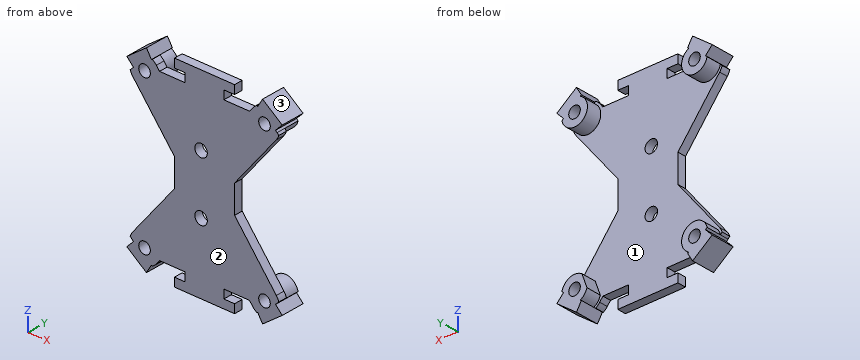
```python
from build123d import *

# Parameters (mm, degrees)
SKETCH1_R               = 24.07
BOSS_EXTRUDE1_DEPTH     = 2
BOSS_EXTRUDE2_DEPTH     = 5.5
BOSS_EXTRUDE5_REACH     = 36.482
SKETCH2_R               = 3
SKETCH1_5_R             = 34.31362745
CUT_EXTRUDE3_DEPTH      = 35.48158639
CUT_EXTRUDE3_DEPTH_BACK = 35.48158639
M2_5_CLEARANCE_HOLE1_D  = 2.7
CUT_EXTRUDE4_DEPTH      = 35.48158639
SKETCH10_R              = 1.45
CUT_EXTRUDE6_DEPTH      = 30.773984948
CUT_EXTRUDE7_DEPTH      = 3.5


with BuildPart() as part:
    # Sketch1 → Boss-Extrude1 (new body)
    with BuildSketch(Plane(origin=(0, 0, 0), x_dir=(1, 0, 0), z_dir=(0, 1, 0))):
        with Locations(Location((0, 0, 0), (0, 0, 270))):
            Circle(SKETCH1_R)
    extrude(amount=BOSS_EXTRUDE1_DEPTH)

    # Sketch1<3> → Boss-Extrude2 (add)
    with BuildSketch(Plane(origin=(0, 0, 0), x_dir=(1, 0, 0), z_dir=(0, 1, 0))):
        with BuildLine():
            ThreePointArc((12.366915807, 20.650043424), (14.541516735, 19.180959075), (16.543257949, 17.483864459))
            Line((16.543257949, 17.483864459), (18.089781085, 19.118318867))
            Line((18.089781085, 19.118318867), (13.523019488, 22.580483607))
            Line((13.523019488, 22.580483607), (12.366915807, 20.650043424))
        make_face()
        with BuildLine():
            ThreePointArc((16.543257949, -17.483864459), (14.541516735, -19.180959075), (12.366915807, -20.650043424))
            Line((12.366915807, -20.650043424), (13.523019488, -22.580483607))
            Line((13.523019488, -22.580483607), (18.089781085, -19.118318867))
            Line((18.089781085, -19.118318867), (16.543257949, -17.483864459))
        make_face()
        with BuildLine():
            ThreePointArc((-16.543257949, 17.483864459), (-14.541516735, 19.180959075), (-12.366915807, 20.650043424))
            Line((-12.366915807, 20.650043424), (-13.523019488, 22.580483607))
            Line((-13.523019488, 22.580483607), (-18.089781085, 19.118318867))
            Line((-18.089781085, 19.118318867), (-16.543257949, 17.483864459))
        make_face()
        with BuildLine():
            ThreePointArc((-12.366915807, -20.650043424), (-14.541516735, -19.180959075), (-16.543257949, -17.483864459))
            Line((-16.543257949, -17.483864459), (-18.089781085, -19.118318867))
            Line((-18.089781085, -19.118318867), (-13.523019488, -22.580483607))
            Line((-13.523019488, -22.580483607), (-12.366915807, -20.650043424))
        make_face()
    extrude(amount=BOSS_EXTRUDE2_DEPTH)

    # Boss-Extrude5: up to this face of the body (flat: up to its plane)
    boss_extrude5_end = Plane(part.part.faces().sort_by_distance((15.168468653, 5.5, 20.00793877))[0])
    # Sketch2 → Boss-Extrude5 (add, up to the picked face)
    with BuildSketch(Plane(origin=(0, 0, 0), x_dir=(1, 0, 0), z_dir=(0, 1, 0)), mode=Mode.PRIVATE) as boss_extrude5_sk1:
        with Locations((13.97, 17.78)):
            Circle(SKETCH2_R)
    boss_extrude5_tool1 = split(extrude(boss_extrude5_sk1.sketch, amount=BOSS_EXTRUDE5_REACH, mode=Mode.PRIVATE), bisect_by=boss_extrude5_end, keep=Keep.BOTH, mode=Mode.PRIVATE)
    # Sketch2 → Boss-Extrude5 (add, up to the picked face)
    with BuildSketch(Plane(origin=(0, 0, 0), x_dir=(1, 0, 0), z_dir=(0, 1, 0)), mode=Mode.PRIVATE) as boss_extrude5_sk2:
        with Locations((13.97, -17.78)):
            Circle(SKETCH2_R)
    boss_extrude5_tool2 = split(extrude(boss_extrude5_sk2.sketch, amount=BOSS_EXTRUDE5_REACH, mode=Mode.PRIVATE), bisect_by=boss_extrude5_end, keep=Keep.BOTH, mode=Mode.PRIVATE)
    # Sketch2 → Boss-Extrude5 (add, up to the picked face)
    with BuildSketch(Plane(origin=(0, 0, 0), x_dir=(1, 0, 0), z_dir=(0, 1, 0)), mode=Mode.PRIVATE) as boss_extrude5_sk3:
        with Locations((-13.97, -17.78)):
            Circle(SKETCH2_R)
    boss_extrude5_tool3 = split(extrude(boss_extrude5_sk3.sketch, amount=BOSS_EXTRUDE5_REACH, mode=Mode.PRIVATE), bisect_by=boss_extrude5_end, keep=Keep.BOTH, mode=Mode.PRIVATE)
    # Sketch2 → Boss-Extrude5 (add, up to the picked face)
    with BuildSketch(Plane(origin=(0, 0, 0), x_dir=(1, 0, 0), z_dir=(0, 1, 0)), mode=Mode.PRIVATE) as boss_extrude5_sk4:
        with Locations((-13.97, 17.78)):
            Circle(SKETCH2_R)
    boss_extrude5_tool4 = split(extrude(boss_extrude5_sk4.sketch, amount=BOSS_EXTRUDE5_REACH, mode=Mode.PRIVATE), bisect_by=boss_extrude5_end, keep=Keep.BOTH, mode=Mode.PRIVATE)
    add(boss_extrude5_tool1.solids().sort_by(Axis((13.97, 0, -17.78), (0, 1, 0)))[0])
    add(boss_extrude5_tool2.solids().sort_by(Axis((13.97, 0, 17.78), (0, 1, 0)))[0])
    add(boss_extrude5_tool3.solids().sort_by(Axis((-13.97, 0, 17.78), (0, 1, 0)))[0])
    add(boss_extrude5_tool4.solids().sort_by(Axis((-13.97, 0, -17.78), (0, 1, 0)))[0])

    # Sketch1<5> → Cut-Extrude3 (cut, two sides)
    with BuildSketch(Plane(origin=(0, 0, 0), x_dir=(1, 0, 0), z_dir=(0, 1, 0))) as cut_extrude3_sk:
        Circle(SKETCH1_5_R)
        with BuildLine():
            Line((18.089781085, 19.118318867), (16.543257949, 17.483864459))
            ThreePointArc((16.543257949, 17.483864459), (22.108382108, 9.517580605), (24.07, 0))
            ThreePointArc((24.07, 0), (22.108382108, -9.517580605), (16.543257949, -17.483864459))
            Line((16.543257949, -17.483864459), (18.089781085, -19.118318867))
            Line((18.089781085, -19.118318867), (13.523019488, -22.580483607))
            Line((13.523019488, -22.580483607), (12.366915807, -20.650043424))
            ThreePointArc((12.366915807, -20.650043424), (0, -24.07), (-12.366915807, -20.650043424))
            Line((-12.366915807, -20.650043424), (-13.523019488, -22.580483607))
            Line((-13.523019488, -22.580483607), (-18.089781085, -19.118318867))
            Line((-18.089781085, -19.118318867), (-16.543257949, -17.483864459))
            ThreePointArc((-16.543257949, -17.483864459), (-24.07, 0), (-16.543257949, 17.483864459))
            Line((-16.543257949, 17.483864459), (-18.089781085, 19.118318867))
            Line((-18.089781085, 19.118318867), (-13.523019488, 22.580483607))
            Line((-13.523019488, 22.580483607), (-12.366915807, 20.650043424))
            ThreePointArc((-12.366915807, 20.650043424), (0, 24.07), (12.366915807, 20.650043424))
            Line((12.366915807, 20.650043424), (13.523019488, 22.580483607))
            Line((13.523019488, 22.580483607), (18.089781085, 19.118318867))
        make_face(mode=Mode.SUBTRACT)
    extrude(amount=CUT_EXTRUDE3_DEPTH, mode=Mode.SUBTRACT)
    extrude(cut_extrude3_sk.sketch, amount=-CUT_EXTRUDE3_DEPTH_BACK, mode=Mode.SUBTRACT)

    # M2.5 Clearance Hole1 (through all)
    with Locations(Plane(origin=(0, 5.5, 0), x_dir=(1, 0, 0), z_dir=(0, 1, 0))):
        with Locations((-13.97, 17.78), (13.97, 17.78), (13.97, -17.78), (-13.97, -17.78)):
            Hole(M2_5_CLEARANCE_HOLE1_D / 2)

    # Sketch8 → Cut-Extrude4 (cut, through all)
    with BuildSketch(Plane.XZ):
        with BuildLine():
            ThreePointArc((-12.157407277, 20.77407876), (-11.650071144, 20.400673597), (-11.217885814, 19.942375432))
            Line((-11.217885814, 19.942375432), (-10.477447975, 19))
            Line((-10.477447975, 19), (-4.5, 19))
            Line((-4.5, 19), (-4.5, 21))
            Line((-4.5, 21), (-7, 21))
            Line((-7, 21), (-7, 23))
            Line((-7, 23), (7, 23))
            Line((7, 23), (7, 21))
            Line((7, 21), (4.5, 21))
            Line((4.5, 21), (4.5, 19))
            Line((4.5, 19), (10.477447975, 19))
            Line((10.477447975, 19), (11.217885814, 19.942375432))
            ThreePointArc((11.217885814, 19.942375432), (11.650071144, 20.400673597), (12.157407277, 20.77407876))
            ThreePointArc((12.157407277, 20.77407876), (0, 24.07), (-12.157407277, 20.77407876))
        make_face()
        with BuildLine():
            Line((7, 3.244024695), (7, -3.244024695))
            Line((7, -3.244024695), (16.722114186, -15.617624568))
            ThreePointArc((16.722114186, -15.617624568), (17.065148682, -16.145969817), (17.307920228, -16.727247155))
            ThreePointArc((17.307920228, -16.727247155), (24.07, 0), (17.307920228, 16.727247155))
            ThreePointArc((17.307920228, 16.727247155), (17.065148682, 16.145969817), (16.722114186, 15.617624568))
            Line((16.722114186, 15.617624568), (7, 3.244024695))
        make_face()
        with BuildLine():
            Line((-7, -3.244024695), (-7, 3.244024695))
            Line((-7, 3.244024695), (-16.722114186, 15.617624568))
            ThreePointArc((-16.722114186, 15.617624568), (-17.065148682, 16.145969817), (-17.307920228, 16.727247155))
            ThreePointArc((-17.307920228, 16.727247155), (-24.07, 0), (-17.307920228, -16.727247155))
            ThreePointArc((-17.307920228, -16.727247155), (-17.065148682, -16.145969817), (-16.722114186, -15.617624568))
            Line((-16.722114186, -15.617624568), (-7, -3.244024695))
        make_face()
        with BuildLine():
            Line((11.217885814, -19.942375432), (10.477447975, -19))
            Line((10.477447975, -19), (4.5, -19))
            Line((4.5, -19), (4.5, -21))
            Line((4.5, -21), (7, -21))
            Line((7, -21), (7, -23))
            Line((7, -23), (-7, -23))
            Line((-7, -23), (-7, -21))
            Line((-7, -21), (-4.5, -21))
            Line((-4.5, -21), (-4.5, -19))
            Line((-4.5, -19), (-10.477447975, -19))
            Line((-10.477447975, -19), (-11.217885814, -19.942375432))
            ThreePointArc((-11.217885814, -19.942375432), (-11.650071144, -20.400673597), (-12.157407277, -20.77407876))
            ThreePointArc((-12.157407277, -20.77407876), (0, -24.07), (12.157407277, -20.77407876))
            ThreePointArc((12.157407277, -20.77407876), (11.650071144, -20.400673597), (11.217885814, -19.942375432))
        make_face()
    extrude(amount=-CUT_EXTRUDE4_DEPTH, mode=Mode.SUBTRACT)

    # Sketch10 → Cut-Extrude6 (cut, through all)
    with BuildSketch(Plane(origin=(0, 0, 0), x_dir=(1, 0, 0), z_dir=(0, 1, 0))):
        with Locations(Location((-0.8, -6.8, 0), (0, 0, 270))):
            Circle(SKETCH10_R)
        with Locations(Location((-0.8, 6.8, 0), (0, 0, 270))):
            Circle(SKETCH10_R)
    extrude(amount=CUT_EXTRUDE6_DEPTH, mode=Mode.SUBTRACT)

    # Sketch11 → Cut-Extrude7 (cut)
    with BuildSketch(Plane(origin=(0, 5.5, 0), x_dir=(1, 0, 0), z_dir=(0, 1, 0))):
        Polygon((0, 0), (17.739781085, 0), (10.209781085, 21), (0, 21), align=None)
    extrude(amount=-CUT_EXTRUDE7_DEPTH, mode=Mode.SUBTRACT)


solid = part.part
```
Here's how the part is built. I have some questions about the finished solid (model axes, mm). Face numbers are marked on the shaded views. Give positions to 0.01 mm unless a question says otherwise; leave off trailing zeros. Write each loop counter-clockwise with the first axis right and the second up, starting at its lowest first coordinate (ties: lowest second). Pieces come first, ordered by that corner, then holes.
(1) Imagine slicing it at D-D, the plane y = 0.95. Count the separate pieces of the cut face and the enclosed holes in it, and give its area (3 significant figures).
Output values:
separate pieces: 1
enclosed holes: 6
area: 1,020 mm2
(2) Imagine slicing it at A-A, the plane x = -0.8. Write out the boundary of the cut face in (y, z), and give its area (3 significant figures).
Output values:
outline: (0, -23) - (2, -23) - (2, -8.25) - (0, -8.25) - close; (0, -5.35) - (2, -5.35) - (2, 5.35) - (0, 5.35) - close; (0, 8.25) - (2, 8.25) - (2, 23) - (0, 23) - close
area: 80.4 mm2
(3) Will these pins go through, and if not, where does the flat tip stop? pin 1 (1 mm diameter, centred on y = 1, z = 20, fed in from -X); pin 2 (2 mm diameter, centred on y = 2, z = 10.5, fed in from -X); pin 3 (0.6 mm diameter, centred on y = 0.5, z = -22, fed in from -X); pin 4 (4.5 mm diameter, centred on x = -13.97, z = 17.78, fed in from +Y).
Output values:
pin 1: stops at x = -17.59
pin 2: stops at x = -13.49
pin 3: stops at x = -14.68
pin 4: stops at y = 5.5
(4) Imagine slicing it at B-B, the plane z = 6.8. Write out the boundary of the cut face in (x, y), and give its area (3 significant figures).
Output values:
outline: (-9.79, 0) - (-2.25, 0) - (-2.25, 2) - (-9.79, 2) - close; (0.65, 0) - (9.79, 0) - (9.79, 2) - (0.65, 2) - close
area: 33.4 mm2
(5) Imagine slicing it at C-C, the plane x = 5. Write out the boundary of the cut face in (y, z), and give its area (3 significant figures).
Output values:
outline: (0, -23) - (2, -23) - (2, -21) - (0, -21) - close; (0, -19) - (2, -19) - (2, 19) - (0, 19) - close; (0, 21) - (2, 21) - (2, 23) - (0, 23) - close
area: 84.0 mm2
(6) If I drill on L1, parallel to Z at x = 13.97, y = 3.2; L2, parallel to Y at x = 2, z = 10; L3, parallel to Z at x = -13.5, y = 3.8, over which ranges is the centre line in solid material (lowest first)?
Output values:
L1: z = -22.24 to -19.13, -16.43 to -14.78, 14.78 to 16.43, 19.13 to 22.24
L2: y = 0 to 2
L3: z = -22.54 to -19.05, -16.51 to -14.82, 14.82 to 16.51, 19.05 to 22.54
(7) Thinking about a two-plate mould opening in X: for the marked faces 1, 2 and 3, which applies, pulls with the +X half, pulls with the -X half, needs draft (parallel to the pull), parting line crosses it, or undercut?
Output values:
face 1: undercut
face 2: needs draft
face 3: pulls with the +X half
